Could you check a few things on this model? Use its own coordinates, in mm. Face numbers are marked on the shaded views. A direction names the side the tool comes from. Coordinates: 2 decimals unless noted, no trailing zeros. Write each loop counter-clockwise with the first axis right and the second up, starting at its lowest first coordinate (ties: lowest second). Pieces come first, ordered by that corner, then holes.
```python
from build123d import *

# Parameters (mm, degrees)
BASEHEAD_DEPTH   = 2
BEARINGFACESKE_W = 0.4
BEARINGFACESKE_H = 0.890426481
FILLET_2_R       = 0.1
THDSCHPAT_COUNT  = 23
THDSCHPAT_PITCH  = 0.5


with BuildPart() as part:
    # BaseHeadSke → BaseHead (new body)
    with BuildSketch(Plane(origin=(0, 0, 0), x_dir=(0, 0, -1), z_dir=(1, 0, 0))):
        Polygon((2.75, 1.58771324), (0, 3.175426481), (-2.75, 1.58771324), (-2.75, -1.58771324), (0, -3.175426481), (2.75, -1.58771324), align=None)
    extrude(amount=BASEHEAD_DEPTH)

    # BodySke → BaseBody (revolve)
    with BuildSketch(Plane.XY, mode=Mode.PRIVATE) as basebody_sk:
        Polygon((0, 0), (14, 0), (14, 1.2195), (13.7195, 1.5), (0, 1.5), align=None)
    revolve(basebody_sk.sketch.rotate(Axis((0, 0, 0), (1, 0, 0)), 90), axis=Axis((0, 0, 0), (1, 0, 0)))

    # HeadChamferSke → HeadChamfer (revolve, cut)
    with BuildSketch(Plane.XY):
        Polygon((0.245620093, 3.175426481), (0, 3.175426481), (0, 2.75), align=None)
    revolve(axis=Axis((0, 0, 0), (1, 0, 0)), mode=Mode.SUBTRACT)

    # BearingFaceSke → BearingFace (revolve, cut)
    with BuildSketch(Plane.XY, mode=Mode.PRIVATE) as bearingface_sk:
        with Locations((1.8, 2.730213241)):
            Rectangle(BEARINGFACESKE_W, BEARINGFACESKE_H)
    revolve(bearingface_sk.sketch.rotate(Axis((0, 0, 0), (1, 0, 0)), 90), axis=Axis((0, 0, 0), (1, 0, 0)), mode=Mode.SUBTRACT)

    # Fillet 2
    fillet_2_edges = [part.edges().sort_by_distance(p)[0] for p in [
        (2, 0, -1.5),
    ]]
    fillet(fillet_2_edges, radius=FILLET_2_R)

    # ThdSchSke → ThreadSchematic (revolve, cut)
    with BuildSketch(Plane.XY, mode=Mode.PRIVATE) as threadschematic_sk:
        Polygon((13.338053249, 1.823893501), (13.338053249, 1.5), (13.5, 1.2195), (13.661946751, 1.5), (13.661946751, 1.823893501), align=None)
    threadschematic = revolve(threadschematic_sk.sketch.rotate(Axis((0, 0, 0), (1, 0, 0)), 90), axis=Axis((0, 0, 0), (1, 0, 0)), mode=Mode.SUBTRACT)

    # ThdSchPat: ThreadSchematic ×23
    with Locations(*[(-i * THDSCHPAT_PITCH, 0, 0) for i in range(1, THDSCHPAT_COUNT)]):
        add(threadschematic, mode=Mode.SUBTRACT)


solid = part.part
```
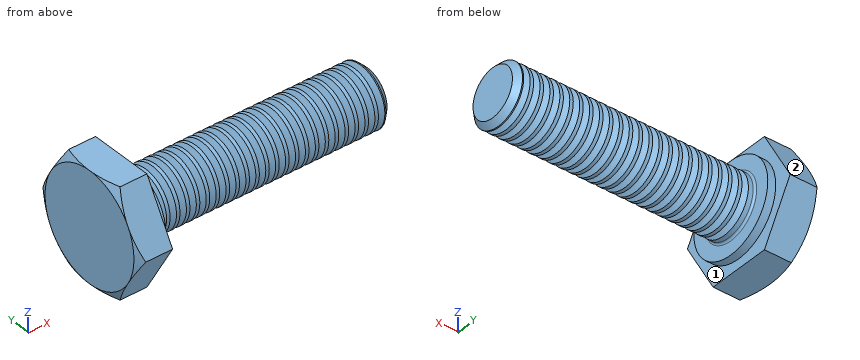
1. On a 3-axis mill with a long thin cutter (end or side, diameter ignored), from which of +Z, -Z, +X, -X, +Y, -Y can I reach the whole of each face in a straight line? I mean the marked faces 1 and 2. Say none if no direction works.
Verdict:
face 1: +X
face 2: +Z, +X, -X, +Y
2. Please list where these lines run through material, in increasing order: line 1 along X through (y, z) = (1, -1.65); line 2 along X through (y, z) = (-1, 2.25); line 3 along Z through (x, y) = (9.75, 0.25).
Verdict:
line 1: x = 0 to 2
line 2: x = 0 to 1.6
line 3: z = -1.48 to 1.48
3. I want a section at A-A on x = 1. Please give me the cut outline in (y, z).
Verdict:
outline: (-3.18, 0) - (-1.59, -2.75) - (1.59, -2.75) - (3.18, 0) - (1.59, 2.75) - (-1.59, 2.75) - close
4. For pin 1 (2 mm diameter, centred on x = 4.5, y = 1.5, fed in from -Z); pin 2 (3 mm diameter, centred on x = 11, y = -0.5, fed in from -Z), each with a flat end and sliding along its axis, tell me the tip position at first contact or that it passes through.
Verdict:
pin 1: stops at z = -1.41
pin 2: stops at z = -1.5
